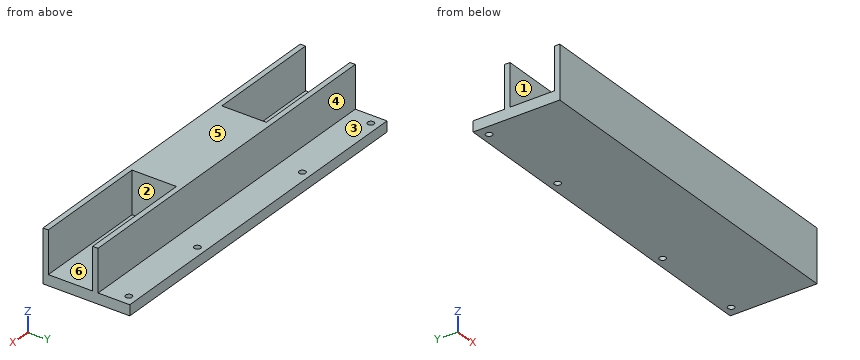
```python
from build123d import *

# Parameters (mm, degrees)
SKETCH_1_W          = 169
SKETCH_1_H          = 41
EXTRUDE_2_DEPTH     = 5
SKETCH_3_R          = 1.5
CUT_EXTRUDE_1_DEPTH = 5
SKETCH_4_W          = 169
SKETCH_4_H          = 26
EXTRUDE_3_DEPTH     = 20
SKETCH_5_W          = 20
SKETCH_5_H          = 21
CUT_EXTRUDE_2_DEPTH = 55
SKETCH_6_W          = 20
SKETCH_6_H          = 21
CUT_EXTRUDE_3_DEPTH = 55


with BuildPart() as part:
    # Эскиз1 → Бобышка-Вытянуть2 (new body)
    with BuildSketch(Plane.XY):
        Rectangle(SKETCH_1_W, SKETCH_1_H)
    extrude(amount=EXTRUDE_2_DEPTH)

    # Эскиз3 → Вырез-Вытянуть1 (cut)
    with BuildSketch(Plane.XY.offset(5)):
        with Locations((79.5, 16.5)):
            Circle(SKETCH_3_R)
        with Locations((34.5, 16.5)):
            Circle(SKETCH_3_R)
        with Locations((-34.5, 16.5)):
            Circle(SKETCH_3_R)
        with Locations((-79.5, 16.5)):
            Circle(SKETCH_3_R)
    extrude(amount=-CUT_EXTRUDE_1_DEPTH, mode=Mode.SUBTRACT)

    # Эскиз4 → Бобышка-Вытянуть3 (add)
    with BuildSketch(Plane.XY.offset(5)):
        with Locations((0, -7.5)):
            Rectangle(SKETCH_4_W, SKETCH_4_H)
    extrude(amount=EXTRUDE_3_DEPTH)

    # Эскиз5 → Вырез-Вытянуть2 (cut)
    with BuildSketch(Plane.ZY.offset(84.5)):
        with Locations((15, -7.5)):
            Rectangle(SKETCH_5_W, SKETCH_5_H)
    extrude(amount=-CUT_EXTRUDE_2_DEPTH, mode=Mode.SUBTRACT)

    # Эскиз6 → Вырез-Вытянуть3 (cut)
    with BuildSketch(Plane(origin=(84.5, 0, 0), x_dir=(0, 0, -1), z_dir=(1, 0, 0))):
        with Locations((-15, -7.5)):
            Rectangle(SKETCH_6_W, SKETCH_6_H)
    extrude(amount=-CUT_EXTRUDE_3_DEPTH, mode=Mode.SUBTRACT)


solid = part.part
```
Design review of the part built by this model. Coordinates are the model's own, in mm. Face numbers are marked on the shaded views. A direction names the side the tool comes from. Give positions to 0.01 mm unless a question says otherwise; leave off trailing zeros. Order: outer loops, then holes, each group sorted by start corner. A loop starts at its lowest first (then second) coordinate and runs counter-clockwise, first axis right, second up. Notation, with made-up numbers: (6.5, -1.5) -> (33.5, -1.5) arc R21 ccw to (33.5, 8.5) -> close; hole circle Ø11 at (-6.5, -32.75). An arc over 180 degrees is marked (long way). Write item = value, one per line. Start each with the question number.
(1) For pin 1 (6 mm diameter, centred on x = 19, z = 19, fed in from +Y); pin 2 (6.5 mm diameter, centred on x = 63, y = -6, fed in from +Z); pin 3 (6 mm diameter, centred on y = -5, z = 14.5, fed in from -X); pin 4 (1.8 mm diameter, centred on x = 34.5, y = 16.5, fed in from -Z), all flat-tipped, find the tip position at first contact; note any pin that passes through.
(2) Mouldability with a two-part tool opening along Y and no side actions: class the marked faces 4, 5 and 6 as +Y half, -Y half, draft (parallel to the pull), parting line (faces both ways), or undercut.
(3) We need section B-B on x = 79.5. Write out the cut boundary in (y, z), plus the area to 3 significant figures.
(4) We need section D-D on y = -3. Write out the cut boundary in (x, z), plus the area to 4 significant figures.
(5) To check wall thickness, follow line 1 along Y through (x, z) = (-52.5, 21); line 2 along Y through (x, z) = (-79.5, 2.4); line 3 along Z through (x, y) = (68.5, -2). State the ranges of each line that lie inside material, in increasing order.
(6) We need section A-A on y = 16.5. Write out the cut boundary in (x, z).
(7) We need section C-C on z = 16.5. Write out the cut boundary in (x, y).
(8) For the marked faces 1, 2 and 3, list the 3-axis set-ups (+Z, -Z, +X, -X, +Y, -Y) from which the entire face can be reached by the end or side of a thin tool; tool diameter is ignored.
Numbers:
q1.pin_1 = 5.5
q1.pin_2 = 5
q1.pin_3 = -29.5
q1.pin_4 = through
q2.face_4 = +Y half
q2.face_5 = draft
q2.face_6 = undercut
q3.outline = (-20.5, 0) -> (15, 0) -> (15, 5) -> (5.5, 5) -> (5.5, 25) -> (3, 25) -> (3, 5) -> (-18, 5) -> (-18, 25) -> (-20.5, 25) -> close; (18, 0) -> (20.5, 0) -> (20.5, 5) -> (18, 5) -> close
q3.area = 290 mm^2
q4.outline = (-84.5, 0) -> (84.5, 0) -> (84.5, 5) -> (29.5, 5) -> (29.5, 25) -> (-29.5, 25) -> (-29.5, 5) -> (-84.5, 5) -> close
q4.area = 2,025 mm^2
q5.line_1 = -20.5 to -18, 3 to 5.5
q5.line_2 = -20.5 to 15, 18 to 20.5
q5.line_3 = 0 to 5
q6.outline = (-84.5, 0) -> (-81, 0) -> (-81, 5) -> (-84.5, 5) -> close; (-78, 0) -> (-36, 0) -> (-36, 5) -> (-78, 5) -> close; (-33, 0) -> (33, 0) -> (33, 5) -> (-33, 5) -> close; (36, 0) -> (78, 0) -> (78, 5) -> (36, 5) -> close; (81, 0) -> (84.5, 0) -> (84.5, 5) -> (81, 5) -> close
q7.outline = (-84.5, -20.5) -> (84.5, -20.5) -> (84.5, -18) -> (29.5, -18) -> (29.5, 3) -> (84.5, 3) -> (84.5, 5.5) -> (-84.5, 5.5) -> (-84.5, 3) -> (-29.5, 3) -> (-29.5, -18) -> (-84.5, -18) -> close
q8.face_1 = +Z, -X
q8.face_2 = +Z, +X
q8.face_3 = +Z, +X, -X, +Y
